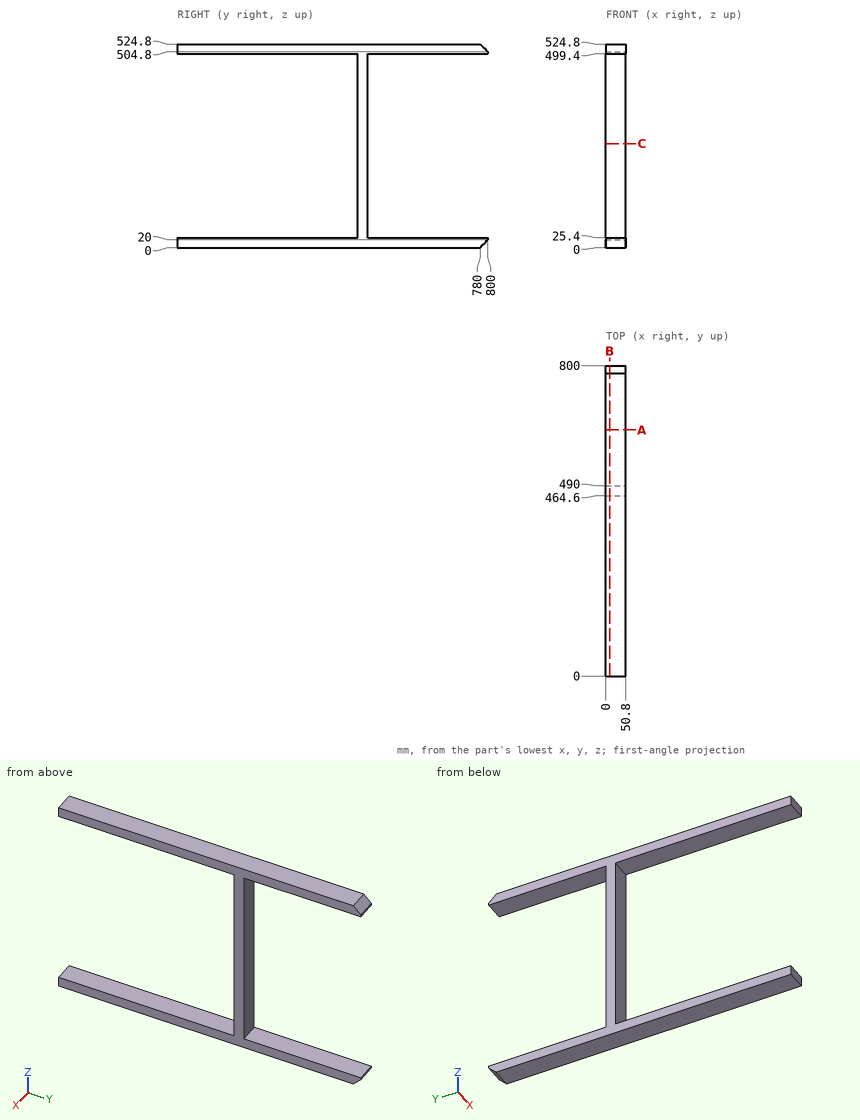
Here's the drawing with two shaded views (mm, measured from the low corner). I have some questions. Round coordinates to 2 decimals unless told otherwise and drop trailing zeros. Order: outer loops, then holes, each group sorted by start corner. A loop starts at its lowest first (then second) coordinate and runs counter-clockwise, first axis right, second up. Notation, with made-up numbers: (88.25, -3) -> (106.25, -3) arc R29 cw to (106.25, 21) -> close; hole circle Ø10 at (-27.5, 7). An arc over 180 degrees is marked (long way). Return JSON: item names as keys, results as strings.
Q1. I need wall thicknesses on line 1 along Z through (x, y) = (13.5, 143); line 2 along Y through (x, z) = (12, 394). Which ranges of each line are inside material? Lowest first, please. Write a range as from..to.
Filled sheet:
{"line 1": "z = 0..25.4, 499.4..524.8", "line 2": "y = 464.6..490"}
Q2. If we section it at B-B on x = 10: List the corners of the cut face in (y, z) for me.
Filled sheet:
{"outline": "(0, 0) -> (780, 0) -> (800, 20) -> (800, 25.4) -> (490, 25.4) -> (490, 499.4) -> (800, 499.4) -> (800, 504.8) -> (780, 524.8) -> (0, 524.8) -> (0, 499.4) -> (464.6, 499.4) -> (464.6, 25.4) -> (0, 25.4) -> close"}
Q3. For pin 1 Ø1.5 at (x, z) = (35, 355.5) entering from -Y, with a flat end and sliding along its axis, tell me the tip position at first contact or that it passes through.
Filled sheet:
{"pin 1": "stops at y = 464.6"}
Q4. If we section it at A-A on y = 634.5: List the corners of the cut face in (x, z) for me.
Filled sheet:
{"outline": "(0, 0) -> (50.8, 0) -> (50.8, 25.4) -> (0, 25.4) -> close; (0, 499.4) -> (50.8, 499.4) -> (50.8, 524.8) -> (0, 524.8) -> close"}
Q5. If we section it at C-C on z = 268: List the corners of the cut face in (x, y) for me, plus the area to 3 significant figures.
Filled sheet:
{"outline": "(0, 464.6) -> (50.8, 464.6) -> (50.8, 490) -> (0, 490) -> close", "area": "1,290 mm^2"}
